For this review, take the finished solid that the model builds, in its own axes (mm). Give positions to 0.01 mm unless a question says otherwise; leave off trailing zeros. Write each loop counter-clockwise with the first axis right and the second up, starting at its lowest first coordinate (ties: lowest second). Pieces come first, ordered by that corner, then holes.
Q1. For line 1 (Y direction, x = 0, z = 2.75); line 2 (X direction, y = -0.5, z = 5.25), list the stretches that pass through material, from the lowest coordinate up.
Q2. We need section A-A (x = 0). Write out the cut boundary in (y, z), then the cut area to 3 significant figures.
Q3. Insertion check: P1, Ø4, axis at y = 2.5, z = 7, coming from the +X side; P2, Ø1, axis at x = -5, z = 1.5, coming from the +Y side; P3, Ø2, axis at x = 4.95, y = -4.95, coming from the +Z side; P4, Ø2, axis at y = -8, z = 4.5, coming from the +X side. Each pin has a flat end and moves straight along its axis. Give the tip position at first contact, or say it passes through.
Q4. We need section C-C (y = 4.25). Write out the cut boundary in (x, z).
Q5. We need section B-B (y = 1.5). Write out the cut boundary in (x, z), then the cut area to 3 significant figures.
Q6. We need section D-D (z = 7.25). Give the number of separate pieces and of enclosed holes in the cut face, then the cut area to 3 significant figures.
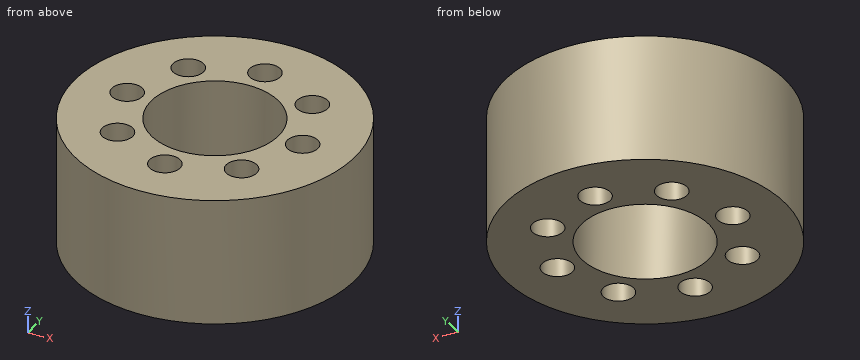
```python
from build123d import *

# Parameters (mm, degrees)
ESQUISSE1_R          = 11
ESQUISSE1_R_2        = 5
BOSS_EXTRU_1_DEPTH   = 10
D_GAGEMENT_M21_D     = 2.4
D_GAGEMENT_M21_DEPTH = 10


with BuildPart() as part:
    # Esquisse1 → Boss.-Extru.1 (new body)
    with BuildSketch(Plane.XY):
        Circle(ESQUISSE1_R)
        Circle(ESQUISSE1_R_2, mode=Mode.SUBTRACT)
    extrude(amount=BOSS_EXTRU_1_DEPTH)

    # Dégagement M21
    with Locations(Plane.XY.offset(10)):
        with Locations((0, 7), (4.949747468, 4.949747468), (7, 0), (4.949747468, -4.949747468), (0, -7), (-4.949747468, -4.949747468), (-7, 0), (-4.949747468, 4.949747468), (0, 0)):
            Hole(D_GAGEMENT_M21_D / 2, depth=D_GAGEMENT_M21_DEPTH)


solid = part.part
```
Computed:
1. line 1: y = -11 to -8.2, -5.8 to -5, 5 to 5.8, 8.2 to 11
1. line 2: x = -10.99 to -8.09, -5.91 to -4.97, 4.97 to 5.91, 8.09 to 10.99
2. outline: (-11, 0) - (-8.2, 0) - (-8.2, 10) - (-11, 10) - close; (-5.8, 0) - (-5, 0) - (-5, 10) - (-5.8, 10) - close; (5, 0) - (5.8, 0) - (5.8, 10) - (5, 10) - close; (8.2, 0) - (11, 0) - (11, 10) - (8.2, 10) - close
2. area: 72.0 mm2
3. P1: stops at x = 10.99
3. P2: stops at y = 10.04
3. P3: passes through
3. P4: stops at x = 8.49
4. outline: (-10.15, 0) - (-5.92, 0) - (-5.92, 10) - (-10.15, 10) - close; (-3.97, 0) - (-2.63, 0) - (-2.63, 10) - (-3.97, 10) - close; (2.63, 0) - (3.97, 0) - (3.97, 10) - (2.63, 10) - close; (5.92, 0) - (10.15, 0) - (10.15, 10) - (5.92, 10) - close
5. outline: (-10.9, 0) - (-4.77, 0) - (-4.77, 10) - (-10.9, 10) - close; (4.77, 0) - (10.9, 0) - (10.9, 10) - (4.77, 10) - close
5. area: 123 mm2
6. separate pieces: 1
6. enclosed holes: 9
6. area: 265 mm2
